Answer from the drawing. Dimensions are ordinates in mm from the lowest x, y and z of the part. Coordinates: 2 decimals unless noted, no trailing zeros. Order: outer loops, then holes, each group sorted by start corner. A loop starts at its lowest first (then second) coordinate and runs counter-clockwise, first axis right, second up. Notation, with made-up numbers: (58, -35) -> (76, -35) arc R24 ccw to (76, -16) -> close; hole circle Ø2 at (-21.5, 49). An arc over 180 degrees is marked (long way). Answer in a Markdown table with one row per item.
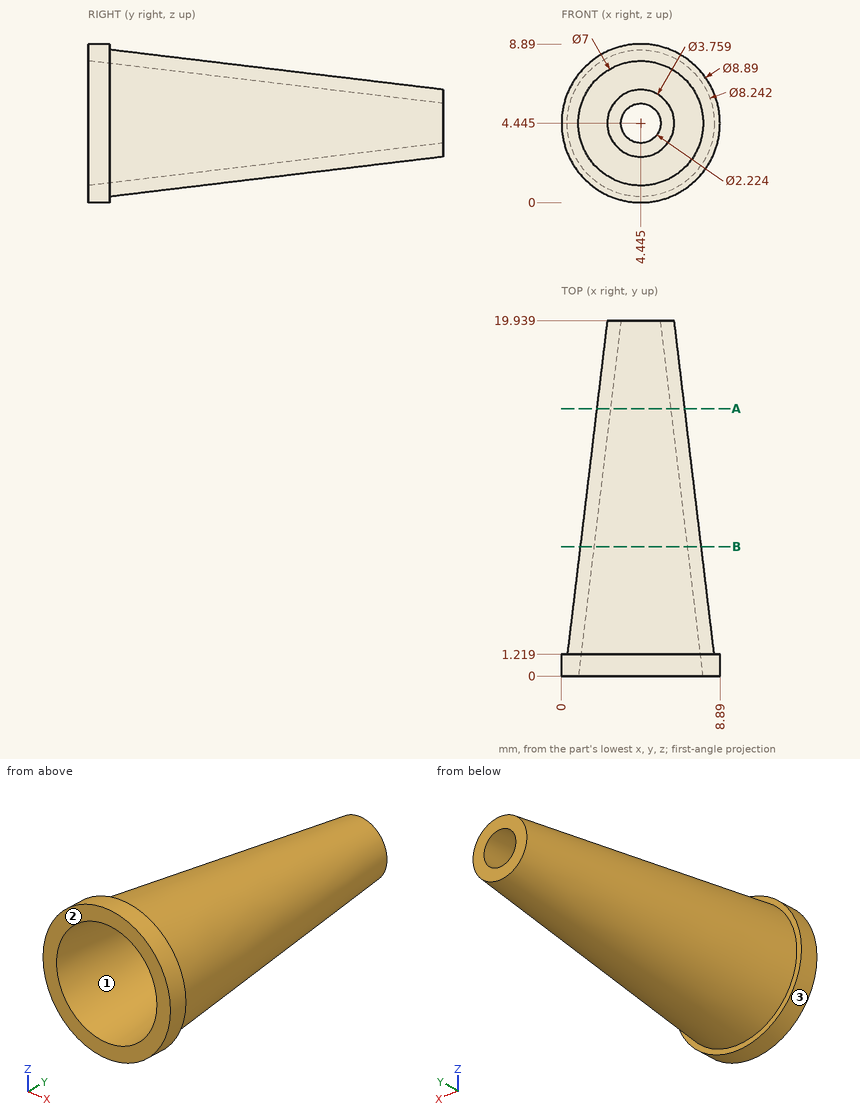
(1) A cutting plane is placed at A-A, the plane y = 15. Determine the outline of the cut face in (x, z) (1 decimal).
Check values:
| item | result |
|---|---|
| outline | circle Ø4.9 at (4.4, 4.4); hole circle Ø3.4 at (4.4, 4.4) |
(2) For a pull along Z with two mould halves and no side action, classify the marked faces 1, 2 and 3 as released by +Z, released by -Z, zero draft, split by the parting line, or undercut.
Check values:
| item | result |
|---|---|
| face 1 | undercut |
| face 2 | zero draft |
| face 3 | split by the parting line |
(3) A cutting plane is placed at B-B, the plane y = 7.25. Determine the outline of the cut face in (x, z) (1 decimal).
Check values:
| item | result |
|---|---|
| outline | circle Ø6.8 at (4.4, 4.4); hole circle Ø5.3 at (4.4, 4.4) |
(4) Find the intervals of material crossed by line 1 along X through (y, z) = (9.25, 4) (1 decimal); line 2 along Z through (x, y) = (5.5, 12.75) (1 decimal); line 3 along X through (y, z) = (17.25, 5.5) (1 decimal), in increasing order. Write a range as from..to.
Check values:
| item | result |
|---|---|
| line 1 | 1.3..2.1, 6.8..7.6 |
| line 2 | 1.9..2.8, 6.1..7 |
| line 3 | 2.5..3.5, 5.4..6.4 |
(5) Flat-ended cylindrical pins translate along their axes: pin 1 (3 mm diameter, centred on x = 6, y = 14, fed in from -Z); pin 2 (5 mm diameter, centred on y = 13, z = 2, fed in from +X); pin 3 (1 mm diameter, centred on y = 4, z = 7, fed in from +X) (1 decimal); pin 4 (4 mm diameter, centred on x = 5, z = 2, fed in from +Y). Find the tip coordinate at first contact, or state that the pin passes through.
Check values:
| item | result |
|---|---|
| pin 1 | z = 1.77 |
| pin 2 | x = 7.3 |
| pin 3 | x = 7.6 |
| pin 4 | y = 19.94 |
